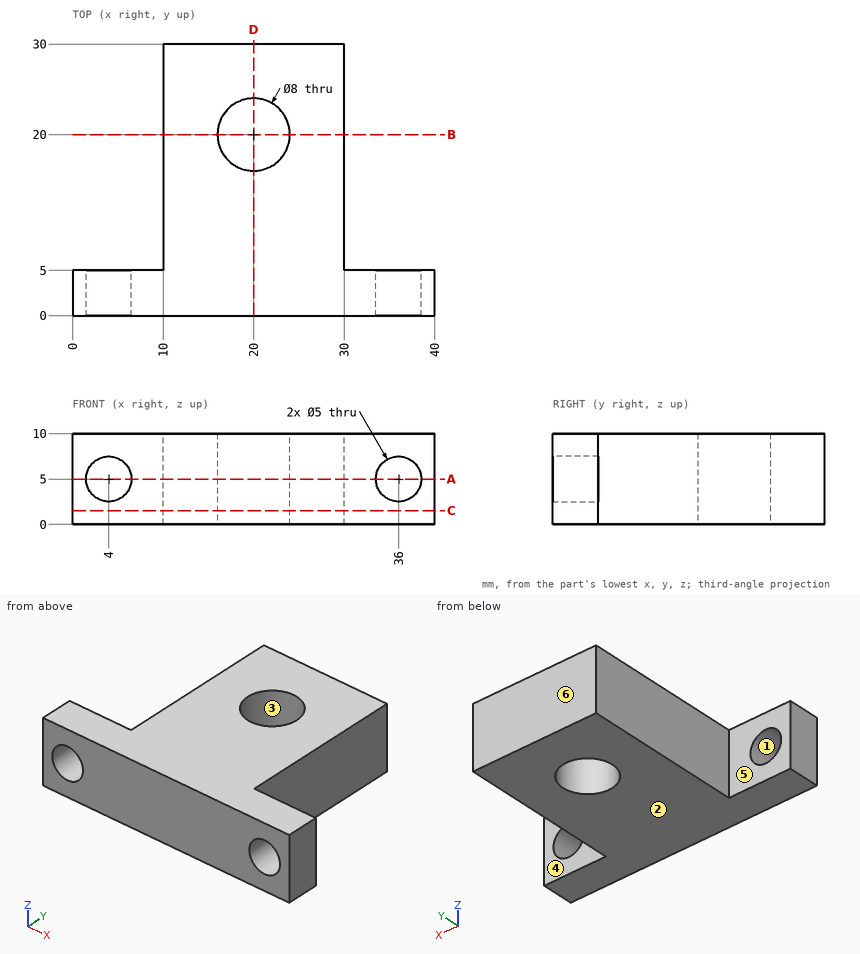
Part print with two shaded views. Sizes in mm from the minimum x, y, z corner. A direction names the side the tool comes from. Give positions to 0.01 mm unless a question says otherwise; leave off trailing zeros. Loops run counter-clockwise (first coordinate to the right, second up) from the corner with the lowest first, then second, coordinate; pieces in that order, holes last. Notation, with made-up numbers: (38.25, -35.75) - (43.25, -35.75) arc R23 cw to (43.25, -12.75) - close; hole circle Ø5 at (66, 64.5). An arc over 180 degrees is marked (long way). Put each result on its own line as item: value.
Q1. Slice it at A-A (z = 5). Give the cut face in (x, y).
Filled in:
outline: (0, 0) - (1.5, 0) - (1.5, 5) - (0, 5) - close; (6.5, 0) - (33.5, 0) - (33.5, 5) - (30, 5) - (30, 30) - (10, 30) - (10, 5) - (6.5, 5) - close; (38.5, 0) - (40, 0) - (40, 5) - (38.5, 5) - close; hole circle Ø8 at (20, 20)
Q2. Tool access for the marked faces 4, 5 and 6: list every direction of +Z, -Z, +X, -X, +Y, -Y with a clear straight run to the whole face (end or side of a thin tool).
Filled in:
face 4: +Z, -Z, +X, +Y
face 5: +Z, -Z, -X, +Y
face 6: +Z, -Z, +X, -X, +Y
Q3. Probe line 1 along X through (y, z) = (2.7, 5); line 2 along Y through (x, z) = (20, 4.75); line 3 along X through (y, z) = (3, 5.75). List the from-to ranges inside material, lowest first.
Filled in:
line 1: x = 0 to 1.5, 6.5 to 33.5, 38.5 to 40
line 2: y = 0 to 16, 24 to 30
line 3: x = 0 to 1.62, 6.38 to 33.62, 38.38 to 40
Q4. Mould opens along Z. For the marked faces 1, 2 and 3 say: pulls with the +Z half, pulls with the -Z half, needs draft (parallel to the pull), parting line crosses it, or undercut.
Filled in:
face 1: undercut
face 2: pulls with the -Z half
face 3: needs draft
Q5. Slice it at B-B (y = 20). Give the cut face in (x, z), plus the area to 3 significant figures.
Filled in:
outline: (10, 0) - (16, 0) - (16, 10) - (10, 10) - close; (24, 0) - (30, 0) - (30, 10) - (24, 10) - close
area: 120 mm²
Q6. Flat gauge pins, fed straight in: pin 1 (1 mm diameter, centred on x = 12.5, y = 5, fed in from -Z); pin 2 (5 mm diameter, centred on y = 12, z = 6, fed in from +X); pin 3 (1.5 mm diameter, centred on y = 14.5, z = 5.5, fed in from -X); pin 4 (3 mm diameter, centred on x = 37.5, z = 6, fed in from +Y). Where does each tip first touch, or does it go through?
Filled in:
pin 1: stops at z = 0
pin 2: stops at x = 30
pin 3: stops at x = 10
pin 4: stops at y = 5
Q7. Slice it at C-C (z = 1.5). Give the cut face in (x, y).
Filled in:
outline: (0, 0) - (40, 0) - (40, 5) - (30, 5) - (30, 30) - (10, 30) - (10, 5) - (0, 5) - close; hole circle Ø8 at (20, 20)
Q8. Slice it at D-D (x = 20). Give the cut face in (y, z).
Filled in:
outline: (0, 0) - (16, 0) - (16, 10) - (0, 10) - close; (24, 0) - (30, 0) - (30, 10) - (24, 10) - close
